```python
from build123d import *

# Parameters (mm, degrees)
SKETCH1_W           = 47
SKETCH1_H           = 23
SKETCH1_R           = 2.5
SKETCH1_R_2         = 1.25
BOSS_EXTRUDE1_DEPTH = 6.35


with BuildPart() as part:
    # Sketch1 → Boss-Extrude1 (new, symmetric)
    with BuildSketch(Plane(origin=(0, 0, 0), x_dir=(1, 0, 0), z_dir=(0, 1, 0))):
        Rectangle(SKETCH1_W, SKETCH1_H)
        with Locations(Location((-10, 0, 0), (0, 0, 270))):
            Circle(SKETCH1_R, mode=Mode.SUBTRACT)
        with Locations(Location((10, 0, 0), (0, 0, 270))):
            Circle(SKETCH1_R, mode=Mode.SUBTRACT)
        with Locations(Location((17.5, 0, 0), (0, 0, 270))):
            Circle(SKETCH1_R_2, mode=Mode.SUBTRACT)
        with Locations(Location((0, 0, 0), (0, 0, 270))):
            Circle(SKETCH1_R_2, mode=Mode.SUBTRACT)
        with Locations(Location((-17.5, 0, 0), (0, 0, 270))):
            Circle(SKETCH1_R_2, mode=Mode.SUBTRACT)
    extrude(amount=BOSS_EXTRUDE1_DEPTH, both=True)


solid = part.part
```
Verification items for the finished model (mm, model axes). Give positions to 0.01 mm unless a question says otherwise; leave off trailing zeros. Loops run counter-clockwise (first coordinate to the right, second up) from the corner with the lowest first, then second, coordinate; pieces in that order, holes last.
1. Section check B-B, the plane x = 10. Enter the section's corners in (y, z), then the cut area to 3 significant figures.
2. Section check A-A, the plane z = 0. Enter the section's corners in (x, y), then the cut area to 3 significant figures.
3. Section check C-C, the plane y = -4.5. Enter the section's corners in (x, z).
4. Mould release check, pull along Z, two halves, no side actions. Record for faces 1 (the flat face through (0, -6.35, -3)), 2 (the cylindrical face through (7.56, -0.09, -0.54)), 3 (the flat face through (0, 0, -11.5)), 4 (the flat face through (0, 0, 11.5)): released by +Z, released by -Z, zero draft, split by the parting line, or undercut.
5. Section check D-D, the plane x = -17.5. Enter the section's corners in (y, z).
6. Thickness scan on line 1 (X direction, y = -3.25, z = 0); line 2 (X direction, y = 2.75, z = -2.25); line 3 (Z direction, x = -8, y = 3.5). Record the ranges inside material, lowest first.
Geometry says:
1. outline: (-6.35, -11.5) - (6.35, -11.5) - (6.35, -2.5) - (-6.35, -2.5) - close; (-6.35, 2.5) - (6.35, 2.5) - (6.35, 11.5) - (-6.35, 11.5) - close
1. area: 229 mm2
2. outline: (-23.5, -6.35) - (-18.75, -6.35) - (-18.75, 6.35) - (-23.5, 6.35) - close; (-16.25, -6.35) - (-12.5, -6.35) - (-12.5, 6.35) - (-16.25, 6.35) - close; (-7.5, -6.35) - (-1.25, -6.35) - (-1.25, 6.35) - (-7.5, 6.35) - close; (1.25, -6.35) - (7.5, -6.35) - (7.5, 6.35) - (1.25, 6.35) - close; (12.5, -6.35) - (16.25, -6.35) - (16.25, 6.35) - (12.5, 6.35) - close; (18.75, -6.35) - (23.5, -6.35) - (23.5, 6.35) - (18.75, 6.35) - close
2. area: 375 mm2
3. outline: (-23.5, -11.5) - (23.5, -11.5) - (23.5, 11.5) - (-23.5, 11.5) - close; hole circle Ø2.5 at (-17.5, 0); hole circle Ø5 at (-10, 0); hole circle Ø2.5 at (0, 0); hole circle Ø5 at (10, 0); hole circle Ø2.5 at (17.5, 0)
4. face 1: zero draft
4. face 2: undercut
4. face 3: released by -Z
4. face 4: released by +Z
5. outline: (-6.35, -11.5) - (6.35, -11.5) - (6.35, -1.25) - (-6.35, -1.25) - close; (-6.35, 1.25) - (6.35, 1.25) - (6.35, 11.5) - (-6.35, 11.5) - close
6. line 1: x = -23.5 to -18.75, -16.25 to -12.5, -7.5 to -1.25, 1.25 to 7.5, 12.5 to 16.25, 18.75 to 23.5
6. line 2: x = -23.5 to -11.09, -8.91 to 8.91, 11.09 to 23.5
6. line 3: z = -11.5 to -1.5, 1.5 to 11.5
